from build123d import *

# Parameters (mm, degrees)
SKETCH1_R           = 114.3
BOSS_EXTRUDE1_DEPTH = 1930.4
SKETCH2_W           = 482.6
SKETCH2_H           = 482.6
BOSS_EXTRUDE2_DEPTH = 152.4


with BuildPart() as part:
    # Sketch1 → Boss-Extrude1 (new body)
    with BuildSketch(Plane(origin=(0, 0, 0), x_dir=(0, 0, -1), z_dir=(1, 0, 0))):
        Circle(SKETCH1_R)
    extrude(amount=BOSS_EXTRUDE1_DEPTH)

    # Sketch2 → Boss-Extrude2 (add)
    with BuildSketch(Plane.ZY):
        Rectangle(SKETCH2_W, SKETCH2_H)
    extrude(amount=BOSS_EXTRUDE2_DEPTH)


solid = part.part
Input: part model. Units: mm. Frame: model coordinates. A direction names the side the tool comes from. Coordinates: 2 decimals unless noted, no trailing zeros. Loops run counter-clockwise (first coordinate to the right, second up) from the corner with the lowest first, then second, coordinate; pieces in that order, holes last. Notation, with made-up numbers: (12.25, -32.5) -> (35.25, -32.5) arc R13 ccw to (35.25, -22.5) -> close; hole circle Ø4 at (59.5, 20.25). An arc over 180 degrees is marked (long way). One line per item, written item: value.
(1) Set-up query: faces 1 (the face through (0, 57, -111)), 2 (the face through (-75, -241.3, -3)). Return all of +Z, -Z, +X, -X, +Y, -Y with unobstructed straight access to the full face (end or side cutting, diameter ignored); none if empty.
Answer below:
face 1: +X
face 2: +Z, -Z, +X, -X, -Y
(2) Cut plane C-C (x = 1781). Output: boundary loops of the cut face in (y, z).
Answer below:
outline: circle Ø228.6 at (0, 0)
(3) Cut plane A-A (z = 0). Output: boundary loops of the cut face in (x, y).
Answer below:
outline: (-152.4, -241.3) -> (0, -241.3) -> (0, -114.3) -> (1930.4, -114.3) -> (1930.4, 114.3) -> (0, 114.3) -> (0, 241.3) -> (-152.4, 241.3) -> close
(4) Cut plane D-D (z = 197.5). Output: boundary loops of the cut face in (x, y), then the cut area to 3 significant figures.
Answer below:
outline: (-152.4, -241.3) -> (0, -241.3) -> (0, 241.3) -> (-152.4, 241.3) -> close
area: 73,500 mm2
(5) Ray query, line 1 along X through (y, z) = (-75, -97); line 2 along Y through (x, z) = (1814.5, 32.5); line 3 along Y through (x, z) = (1696, -62). Return the intervals inside material, ascending.
Answer below:
line 1: x = -152.4 to 0
line 2: y = -109.58 to 109.58
line 3: y = -96.02 to 96.02
(6) Pin query (flat end, axial travel): pin 1 Ø4 at (x, y) = (1479, -70.5) entering from +Z; pin 2 Ø2 at (x, z) = (369, -36.5) entering from +Y; pin 3 Ø4 at (x, z) = (1110.5, -57.5) entering from -Y. Return the tip coordinate at first contact, or that it passes through.
Answer below:
pin 1: stops at z = 91.5
pin 2: stops at y = 108.65
pin 3: stops at y = -99.92
